```python
from build123d import *

# Parameters (mm, degrees)
BOSS_EXTRUDE1_DEPTH = 45
SKETCH2_W           = 20
SKETCH2_H           = 12.5
BOSS_EXTRUDE2_DEPTH = 20
FILLET1_R           = 10
FILLET2_R           = 10
SKETCH3_R           = 5
CUT_EXTRUDE1_DEPTH  = 50
CUT_EXTRUDE2_DEPTH  = 55
SKETCH5_R           = 7.5
CUT_EXTRUDE3_DEPTH  = 55


with BuildPart() as part:
    # Sketch1 → Boss-Extrude1 (new body)
    with BuildSketch(Plane.XY):
        with BuildLine():
            Line((0, 0), (70, 0))
            Line((70, 0), (99.838459525, 29.838459525))
            Line((99.838459525, 29.838459525), (93.338433206, 38.064606978))
            Line((93.338433206, 38.064606978), (58.056372922, 21.612312072))
            ThreePointArc((58.056372922, 21.612312072), (53.393996431, 20.684907727), (48.830190304, 22.015135905))
            Line((48.830190304, 22.015135905), (9.27982655, 44.849549065))
            Line((9.27982655, 44.849549065), (-25.72017345, 44.849549065))
            Line((-25.72017345, 44.849549065), (-25.72017345, 14.849549065))
            Line((-25.72017345, 14.849549065), (0, 0))
        make_face()
    extrude(amount=BOSS_EXTRUDE1_DEPTH)

    # Sketch2 → Boss-Extrude2 (add)
    with BuildSketch(Plane(origin=(0, 44.849549065, 0), x_dir=(1, 0, 0), z_dir=(0, 1, 0))):
        with Locations((-8.22017345, -6.25)):
            Rectangle(SKETCH2_W, SKETCH2_H)
        with Locations((-8.22017345, -38.75)):
            Rectangle(SKETCH2_W, SKETCH2_H)
    extrude(amount=BOSS_EXTRUDE2_DEPTH)

    # Fillet1
    fillet1_edges = [part.edges().sort_by_distance(p)[0] for p in [
        (1.77982655, 64.849549065, 38.75),
        (-18.22017345, 64.849549065, 38.75),
        (1.77982655, 64.849549065, 6.25),
        (-18.22017345, 64.849549065, 6.25),
    ]]
    fillet(fillet1_edges, radius=FILLET1_R - 0.0001)  # a hair under: the kernel refuses the full size

    # Fillet2
    fillet2_edges = [part.edges().sort_by_distance(p)[0] for p in [
        (9.27982655, 44.849549065, 22.5),
    ]]
    fillet(fillet2_edges, radius=FILLET2_R)

    # Sketch3 → Cut-Extrude1 (cut)
    with BuildSketch(Plane.XY.offset(45)):
        with Locations((-8.22017345, 54.849549065)):
            Circle(SKETCH3_R)
    extrude(amount=-CUT_EXTRUDE1_DEPTH, mode=Mode.SUBTRACT)

    # Sketch4 → Cut-Extrude2 (cut)
    with BuildSketch(Plane(origin=(0, 44.849549065, 0), x_dir=(1, 0, 0), z_dir=(0, 1, 0))):
        with BuildLine():
            Line((11.600334626, -17.5), (21.600334626, -17.5))
            ThreePointArc((21.600334626, -17.5), (26.600334626, -22.5), (21.600334626, -27.5))
            Line((21.600334626, -27.5), (11.600334626, -27.5))
            ThreePointArc((11.600334626, -27.5), (6.600334626, -22.5), (11.600334626, -17.5))
        make_face()
    extrude(amount=-CUT_EXTRUDE2_DEPTH, mode=Mode.SUBTRACT)

    # Sketch5 → Cut-Extrude3 (cut)
    with BuildSketch(Plane.XY.offset(45)):
        with Locations((16.77982655, 24.849549065)):
            Circle(SKETCH5_R)
    extrude(amount=-CUT_EXTRUDE3_DEPTH, mode=Mode.SUBTRACT)


solid = part.part
```
CAD build for the part. Positions are in the model's coordinates, mm. A direction names the side the tool comes from. Give positions to 0.01 mm unless a question says otherwise; leave off trailing zeros. Loops run counter-clockwise (first coordinate to the right, second up) from the corner with the lowest first, then second, coordinate; pieces in that order, holes last. Notation, with made-up numbers: (-7.5, 79.5) -> (0.5, 79.5) arc R17 ccw to (0.5, 95.5) -> close; hole circle Ø3 at (-18.75, 9.25). An arc over 180 degrees is marked (long way). Use a Markdown table: item, result.
1. Slice it at A-A (x = 16). List the corners of the cut face in (y, z), plus the area to 3 significant figures.
Check result:
| item | result |
|---|---|
| outline | (0, 0) -> (17.39, 0) -> (17.39, 17.5) -> (0, 17.5) -> close; (0, 27.5) -> (17.39, 27.5) -> (17.39, 45) -> (0, 45) -> close; (32.31, 0) -> (40.97, 0) -> (40.97, 17.5) -> (32.31, 17.5) -> close; (32.31, 27.5) -> (40.97, 27.5) -> (40.97, 45) -> (32.31, 45) -> close |
| area | 912 mm^2 |
2. Which spindle directions (+Z, -Z, +X, -X, +Y, -Y) get a long thin tool onto all of the face, cutting with end or side? Do faces 1 (the flat face through (-18.22, 50, 6)), 2 (the cylindrical face through (-8.871, 59.807, 6.337)), 3 (the flat face through (30.5, 32.6, 22.2)), 4 (the flat face through (17, 10, 17.5)). Say none if no direction does.
Check result:
| item | result |
|---|---|
| face 1 | +Z, -Z, -X, +Y |
| face 2 | +Z, -Z |
| face 3 | +Z, -Z, +Y |
| face 4 | +Y, -Y |
3. Flat gauge pins, fed straight in: pin 1 (1.5 mm diameter, centred on x = -12, y = 20.5, fed in from -Z); pin 2 (11 mm diameter, centred on y = 51, z = 40.5, fed in from -X); pin 3 (5 mm diameter, centred on y = 49.5, z = 39.5, fed in from +X); pin 4 (6 mm diameter, centred on x = 48, z = 14, fed in from +Y). Where does each tip first touch, or does it go through?
Check result:
| item | result |
|---|---|
| pin 1 | stops at z = 0 |
| pin 2 | stops at x = -18.22 |
| pin 3 | stops at x = 1.78 |
| pin 4 | stops at y = 24.23 |
4. Mould opens along X. For faces 5 (the flat face through (-11, 50, 12.5)), 6 (the flat face through (1.78, 50, 39)), 7 (the cylindrical face through (-8.871, 59.807, 38.838)) say: pulls with the +X half, pulls with the -X half, needs draft (parallel to the pull), parting line crosses it, or undercut.
Check result:
| item | result |
|---|---|
| face 5 | needs draft |
| face 6 | pulls with the +X half |
| face 7 | undercut |
5. Slice it at B-B (y = 36). List the corners of the cut face in (x, z), plus the area to 3 significant figures.
Check result:
| item | result |
|---|---|
| outline | (-25.72, 0) -> (24.61, 0) -> (24.61, 18.51) arc R5 cw to (21.6, 17.5) -> (11.6, 17.5) arc R5 cw to (11.6, 27.5) -> (21.6, 27.5) arc R5 cw to (24.61, 26.49) -> (24.61, 45) -> (-25.72, 45) -> close; (88.91, 0) -> (94.97, 0) -> (94.97, 45) -> (88.91, 45) -> close |
| area | 2,370 mm^2 |
6. Slice it at D-D (y = 58.5). List the corners of the cut face in (x, z).
Check result:
| item | result |
|---|---|
| outline | (-17.53, 0) -> (-11.64, 0) -> (-11.64, 12.5) -> (-17.53, 12.5) -> close; (-17.53, 32.5) -> (-11.64, 32.5) -> (-11.64, 45) -> (-17.53, 45) -> close; (-4.8, 0) -> (1.09, 0) -> (1.09, 12.5) -> (-4.8, 12.5) -> close; (-4.8, 32.5) -> (1.09, 32.5) -> (1.09, 45) -> (-4.8, 45) -> close |
7. Slice it at C-C (z = 34). Give the number of separate pieces and of enclosed holes in the cut face, plus the area to 3 significant figures.
Check result:
| item | result |
|---|---|
| separate pieces | 1 |
| enclosed holes | 2 |
| area | 3,820 mm^2 |
8. Wall check: L1, parallel to X at y = 22, z = 26.5; L2, parallel to Y at x = 16, z = 12; L3, parallel to X at y = 48, z = 41.5. Give the ranges that are in metal, low to high. Write a range as [from, to].
Check result:
| item | result |
|---|---|
| L1 | x = [-25.72, 8.6], [24.6, 48.86], [58.89, 92] |
| L2 | y = [0, 17.39], [32.31, 40.97] |
| L3 | x = [-18.22, 1.78] |
